Read the model definition and answer for the solid it produces. Units are mm, in the model's axes. Face numbers are marked on the shaded views. A direction names the side the tool comes from. Coordinates: 2 decimals unless noted, no trailing zeros. Order: outer loops, then holes, each group sorted by start corner. A loop starts at its lowest first (then second) coordinate and runs counter-clockwise, first axis right, second up. Notation, with made-up numbers: M -38,-7.5 L 16,-7.5 A27 cw 16,17.5 Z; hole C -28,-37 d10. An arc over 180 degrees is marked long. Write each question's results on one line, items separated by ' | '.
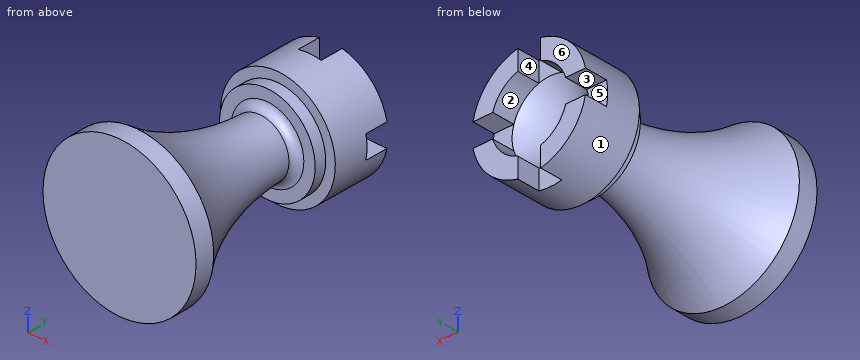
```python
from build123d import *

# Parameters (mm, degrees)
FILLET1_R               = 2
CUT_EXTRUDE1_REACH      = 52.636
CUT_EXTRUDE1_END_RADIUS = 15
SKETCH2_W               = 6
SKETCH2_H               = 12
CIRPATTERN1_COUNT       = 4
SCALE_1_SCALE           = 0.6


with BuildPart() as part:
    # Sketch1 → Revolve1 (revolve)
    with BuildSketch(Plane.XY, mode=Mode.PRIVATE) as revolve1_sk:
        with BuildLine():
            Line((20, -37), (20, -42))
            Line((20, -42), (0, -42))
            Line((0, -42), (0, 0))
            Line((0, 0), (0, 8))
            ThreePointArc((0, 8), (5.346686076, 9.133284811), (10, 12))
            Line((10, 12), (10, 18))
            Line((10, 18), (15, 18))
            Line((15, 18), (15, 3))
            Line((15, 3), (12.5, 3))
            Line((12.5, 3), (12.5, 0))
            Line((12.5, 0), (7.5, 0))
            ThreePointArc((7.5, 0), (10.655312326, -19.545502593), (20, -37))
        make_face()
    revolve(revolve1_sk.sketch.rotate(Axis((0, 46.622291022, 0), (0, -1, 0)), 90), axis=Axis((0, 46.622291022, 0), (0, -1, 0)))

    # Fillet1
    fillet1_edges = [part.edges().sort_by_distance(p)[0] for p in [
        (0, 0, -7.5),
    ]]
    fillet(fillet1_edges, radius=FILLET1_R)

    # Cut-Extrude1: up to this cylinder (the profile starts inside it)
    cut_extrude1_end = Plane(origin=(0, 18, 0), z_dir=(0, 1, 0)) * Cylinder(CUT_EXTRUDE1_END_RADIUS, 136.272, mode=Mode.PRIVATE)
    # Sketch2 → Cut-Extrude1 (cut, up to the surface)
    with BuildSketch(Plane.XY, mode=Mode.PRIVATE) as cut_extrude1_sk1:
        with Locations((0, 18)):
            Rectangle(SKETCH2_W, SKETCH2_H)
    cut_extrude1_tool1 = extrude(cut_extrude1_sk1.sketch, amount=-CUT_EXTRUDE1_REACH, mode=Mode.PRIVATE) & cut_extrude1_end
    cut_extrude1 = cut_extrude1_tool1.solids().sort_by_distance((0, 18, 0))[0]
    add(cut_extrude1, mode=Mode.SUBTRACT)

    # CirPattern1: Cut-Extrude1 ×4 about axis
    cirpattern1_axis = Axis((0, 0, 0), (0, 1, 0))
    for i in range(1, CIRPATTERN1_COUNT):
        add(cut_extrude1.rotate(cirpattern1_axis, i * 360 / CIRPATTERN1_COUNT), mode=Mode.SUBTRACT)


with BuildPart() as part_1:
    # 缩放比例1: scaled about (0, 0, 0)
    add(part.part.scale(SCALE_1_SCALE))


solid = part_1.part
```
(1) The part is cut by section B-B, the plane y = -17. Write down the section's boundary in (x, z).
Conclusion:
outline: C 0,0 d17.31
(2) The mould has two halves that part along X. Classify the marked faces 1, 2 and 3: pulls with the +X half, pulls with the -X half, needs draft (parallel to the pull), parting line crosses it, or undercut.
Conclusion:
face 1: parting line crosses it | face 2: undercut | face 3: needs draft
(3) Straight lines are drawn through the part: line 1 (Z direction, x = 5, y = 9.5); line 2 (X direction, y = 1.5, z = 0.5); line 3 (X direction, y = -10, z = -3.75). For each, find the intervals that lie inside material, in ascending order.
Conclusion:
line 1: -7.48 to -3.32, 3.32 to 7.48 | line 2: -7.48 to 7.48 | line 3: -4.5 to 4.5
(4) For the marked faces 4, 5 and 6, determine the directions among +Z, -Z, +X, -X, +Y, -Y from which every point of the face is accessible in a straight line to the end or side of a thin tool.
Conclusion:
face 4: +Z, -Z, +Y | face 5: +X, -X, +Y | face 6: +Z, -Z, +X, -X, +Y
(5) The part is cut by section A-A, the plane y = 0.5. Write down the section's boundary in (x, z).
Conclusion:
outline: C 0,0 d15
(6) Given pin 1 (0.9 mm diameter, centred on y = 8.5, z = 6.5, fed in from +X); pin 2 (3.5 mm diameter, centred on x = 0, z = 7, fed in from +Y); pin 3 (1.5 mm diameter, centred on y = 8, z = -6.5, fed in from -X), each flat-ended and moving along its own axis, determine where each tip first touches the part or whether it passes through.
Conclusion:
pin 1: x = 6.66 | pin 2: y = 7.2 | pin 3: x = -6.92
